Autodesk Inventor part; units mm, degrees
ref_plane "YZ Plane" through (0, 0, 0) normal (1, 0, 0) x (0, 1, 0)
ref_plane "XZ Plane" through (0, 0, 0) normal (0, 1, 0) x (-1, 0, 0)
ref_plane "XY Plane" through (0, 0, 0) normal (0, 0, 1) x (1, 0, 0)
sketch "Sketch1" plane through (0, 0, 0) normal (0, 0, 1) x (1, 0, 0)
  line L0 (0, 0) -> (40.005, 0)
  line L1 (40.005, 0) -> (40.005, -40.005)
  line L2 (40.005, -40.005) -> (0, -40.005)
  line L3 (0, -40.005) -> (0, 0)
  dimension "d0" = 40.005
  dimension "d1" = 40.005
extrude "Extrusion1" add sketch "Sketch1" along normal blind 10.16
sketch "Sketch2" plane through (0, 0, 10.16) normal (0, 0, 1) x (1, 0, 0)
  line L0 (40.005, 0) -> (0, 0)
  line L1 (0, 0) -> (0, -40.005)
  line L2 (0, -40.005) -> (40.005, -40.005)
  line L3 (40.005, -40.005) -> (40.005, 0)
  circle A0 centre (20.0025, -20.0025) radius 19.05
  circle A1 centre (3.81, -3.81) radius 1.778
  circle A2 centre (36.195, -3.81) radius 1.778
  circle A3 centre (36.195, -36.195) radius 1.778
  circle A4 centre (3.81, -36.195) radius 1.778
  dimension "d4" = 38.1
  dimension "d6" = 3.81
  dimension "d7" = 3.81
  dimension "d8" = 3.81
  dimension "d9" = 3.81
  dimension "d10" = 3.556
  dimension "d11" = 3.556
  dimension "d12" = 3.556
  dimension "d13" = 3.556
extrude "Extrusion2" cut sketch "Sketch2" against normal blind 12.7 contours A0 | A1 | A2 | A3 | A4
sketch "Sketch3" plane through (0, 0, 10.16) normal (0, 0, 1) x (1, 0, 0)
  circle A0 centre (20.0025, -20.0025) radius 19.05
  circle A1 centre (20.0025, -20.0025) radius 10.287
  dimension "d16" = 20.574
extrude "Extrusion3" add sketch "Sketch3" against normal blind 10.16 contours A1
sketch "Sketch4" plane through (40.005, -40.005, 0) normal (1, 0, 0) x (0, 0, -1)
  line L0 (-10.16, 0) -> (-10.16, 40.005)
  line L1 (-10.16, 21.2725) -> (-8.89, 21.2725)
  line L2 (-8.89, 21.2725) -> (-8.89, 18.7325)
  line L3 (-8.89, 18.7325) -> (-10.16, 18.7325)
  line L4 (-10.16, 18.7325) -> (-10.16, 21.2725)
  point P0 (-10.16, 20.0025)
  dimension "d20" = 1.27
  dimension "d21" = 1.27
  dimension "d22" = 1.27
extrude "Extrusion4" add sketch "Sketch4" against normal blind 10.16
chamfer "Chamfer1" distance 2.54 angle 45 4 edges at (0, 0, 5.08) (40.005, 0, 5.08) (40.005, -40.005, 5.08) (0, -40.005, 5.08)
properties part number "Fan"
Source: CAD feature listing. Evaluate the final solid. Frame: model axes, mm. A direction names the side the tool comes from. Give positions to 0.01 mm unless a question says otherwise; leave off trailing zeros. Order: outer loops, then holes, each group sorted by start corner. A loop starts at its lowest first (then second) coordinate and runs counter-clockwise, first axis right, second up.
(1) Access query for faces 5 (the face through (1.252, -38.717, 5.009)), 6 (the face through (35, -18.732, 10)). Directions: +Z, -Z, +X, -X, +Y, -Y. A direction counts if a zero-diameter tool reaches every point of the face in a straight line with its end or side. Return the directions, or none.
(2) Material intervals for line 1 along Y through (x, z) = (24.5, 5.75) (3 decimals); line 2 along Y through (x, z) = (28, 1.5) (3 decimals); line 3 along Y through (x, z) = (3.81, 5) (3 decimals), sorted ascending.
(3) Section query B-B (y = -4.5). Return the cut outline in (x, z) (3 decimals), plus the area to 3 significant figures.
(4) Pull-direction query (X, two-part tool) for faces 1 (the face through (35, -21.272, 10)), 2 (the face through (38.72, -38.75, 5.01)), 3 (the face through (35, -20, 8.89)), 4 (the face through (20, -20, 10.16)); classes: +X half, -X half, draft (parallel to the pull), parting line (faces both ways), or undercut.
(5) Section query A-A (x = 3.81). Return the cut outline in (y, z) (3 decimals), plus the area to 3 significant figures.
(6) Section query C-C (z = 3.5). State how many separate pieces and enclosed holes the cut face has, plus the area to 3 significant figures.
(7) Section query D-D (x = 16). Return the cut outline in (y, z) (3 decimals).
(8) Contact query for a flat-ended pin moving along its axis: P1, Ø3, axis at x = 33.5, y = -20, coming from the -Z side. Output: stop coordinate, or through.
Outcome:
1. face 5: +Z, -Z, -X, -Y
1. face 6: +Z, -Z
2. line 1: y = -40.005 to -38.514, -29.254 to -10.751, -1.491 to 0
2. line 2: y = -40.005 to -37.292, -26.473 to -13.532, -2.713 to 0
2. line 3: y = -40.005 to -37.973, -34.417 to -30.038, -9.967 to -5.588, -2.032 to 0
3. outline: (0, 0) - (2.171, 0) - (2.171, 10.16) - (0, 10.16) - close; (5.449, 0) - (8.931, 0) - (8.931, 10.16) - (5.449, 10.16) - close; (31.074, 0) - (34.556, 0) - (34.556, 10.16) - (31.074, 10.16) - close; (37.834, 0) - (40.005, 0) - (40.005, 10.16) - (37.834, 10.16) - close
3. area: 115 mm2
4. face 1: undercut
4. face 2: +X half
4. face 3: undercut
4. face 4: draft
5. outline: (-40.005, 0) - (-37.973, 0) - (-37.973, 10.16) - (-40.005, 10.16) - close; (-34.417, 0) - (-30.038, 0) - (-30.038, 10.16) - (-34.417, 10.16) - close; (-9.967, 0) - (-5.588, 0) - (-5.588, 10.16) - (-9.967, 10.16) - close; (-2.032, 0) - (0, 0) - (0, 10.16) - (-2.032, 10.16) - close
5. area: 130 mm2
6. separate pieces: 2
6. enclosed holes: 5
6. area: 740 mm2
7. outline: (-40.005, 0) - (-38.627, 0) - (-38.627, 10.16) - (-40.005, 10.16) - close; (-29.479, 0) - (-10.526, 0) - (-10.526, 10.16) - (-29.479, 10.16) - close; (-1.378, 0) - (0, 0) - (0, 10.16) - (-1.378, 10.16) - close
8. P1: stops at z = 8.89
